Source: CAD feature listing. Evaluate the final solid. Frame: model axes, mm. Face numbers are marked on the shaded views. A direction names the side the tool comes from. Round coordinates to 2 decimals unless told otherwise and drop trailing zeros. Loops run counter-clockwise (first coordinate to the right, second up) from the corner with the lowest first, then second, coordinate; pieces in that order, holes last. Notation, with made-up numbers: (85.25, 42) -> (97.25, 42) arc R19 cw to (97.25, 72) -> close; hole circle Ø9 at (-2, -27). An arc over 180 degrees is marked (long way). Put each result on its own line as item: value. Start each with the question number.
1. Cut plane D-D (x = -65.5). Return the cut outline in (y, z), then the cut area to 3 significant figures.
2. Draft query along X for the marked faces 3, 4, 5 and 6. Return one class per face: pulls with the +X half, pulls with the -X half, needs draft (parallel to the pull), parting line crosses it, or undercut.
3. Contact query for flat-ended pins moving along their axis: pin 1 (8 mm diameter, centred on x = 70.5, z = 36, fed in from +Y); pin 2 (2 mm diameter, centred on y = 35.5, z = 20.5, fed in from -X); pin 3 (5 mm diameter, centred on y = 13.5, z = 41.25, fed in from -X). Output: stop coordinate, or through.
4. Cut plane A-A (y = 18). Return the cut outline in (x, z).
5. Cut plane C-C (y = 8.5). Return the cut outline in (x, z), then the cut area to 3 significant figures.
6. Cut plane B-B (x = 39). Return the cut outline in (y, z), then the cut area to 4 significant figures.
7. Material intervals for L1, parallel to Z at x = -115.2, y = 4.5; L2, parallel to Y at x = -14.5, z = 3; L3, parallel to X at y = 10.5, z = 25.5, sorted ascending.
8. Set-up query: the marked faces 1 and 2. Return all of +Z, -Z, +X, -X, +Y, -Y with unobstructed straight access to the full face (end or side cutting, diameter ignored); none if empty.
```python
from build123d import *

# Parameters (mm, degrees)
BOSS_EXTRUDE1_DEPTH     = 45
CUT_EXTRUDE1_DEPTH      = 7.5
SKETCH4_R               = 1.5
CUT_EXTRUDE2_DEPTH      = 7.5
CUT_EXTRUDE3_DEPTH      = 139.338353323
CUT_EXTRUDE3_DEPTH_BACK = 139.338353323
SKETCH5_R               = 1.5


with BuildPart() as part:
    # Sketch1 → Boss-Extrude1 (new body)
    with BuildSketch(Plane.XY):
        with BuildLine():
            ThreePointArc((-112.5, 0), (-97.123106012, 37.123106012), (-60, 52.5))
            Line((-60, 52.5), (60, 52.5))
            ThreePointArc((60, 52.5), (97.123106012, 37.123106012), (112.5, 0))
            Line((112.5, 0), (117.5, 0))
            ThreePointArc((117.5, 0), (100.658639918, 40.658639918), (60, 57.5))
            Line((60, 57.5), (-60, 57.5))
            ThreePointArc((-60, 57.5), (-100.658639918, 40.658639918), (-117.5, 0))
            Line((-117.5, 0), (-112.5, 0))
        make_face()
    extrude(amount=BOSS_EXTRUDE1_DEPTH)

    # Sketch3 → Cut-Extrude1 (cut)
    with BuildSketch(Plane.XY.offset(45)):
        with BuildLine():
            Line((-115.5, 0), (115.5, 0))
            ThreePointArc((115.5, 0), (99.244426356, 39.244426356), (60, 55.5))
            Line((60, 55.5), (-60, 55.5))
            ThreePointArc((-60, 55.5), (-99.244426356, 39.244426356), (-115.5, 0))
        make_face()
    extrude(amount=-CUT_EXTRUDE1_DEPTH, mode=Mode.SUBTRACT)

    # Sketch4 → Cut-Extrude2 (cut)
    with BuildSketch(Plane(origin=(0, 57.5, 0), x_dir=(1, 0, 0), z_dir=(0, 1, 0))):
        with Locations(Location((33, -3.75, 0), (0, 0, 270))):
            Circle(SKETCH4_R)
        with Locations(Location((11, -41.25, 0), (0, 0, 270))):
            Circle(SKETCH4_R)
        with Locations(Location((33, -41.25, 0), (0, 0, 270))):
            Circle(SKETCH4_R)
        with Locations(Location((55, -41.25, 0), (0, 0, 270))):
            Circle(SKETCH4_R)
        with Locations(Location((-33, -3.75, 0), (0, 0, 180))):
            Circle(SKETCH4_R)
        with Locations(Location((-11, -41.25, 0), (0, 0, 180))):
            Circle(SKETCH4_R)
        with Locations(Location((-33, -41.25, 0), (0, 0, 180))):
            Circle(SKETCH4_R)
        with Locations(Location((-55, -41.25, 0), (0, 0, 180))):
            Circle(SKETCH4_R)
    extrude(amount=-CUT_EXTRUDE2_DEPTH, mode=Mode.SUBTRACT)

    # Sketch5 → Cut-Extrude3 (cut, two sides: drawn at the far end of the back side and taken through both)
    with BuildSketch(Plane(origin=(0, 0, 0), x_dir=(0, 0, -1), z_dir=(1, 0, 0)).offset(-CUT_EXTRUDE3_DEPTH_BACK)):
        with Locations((-3.75, 4.5)):
            Circle(SKETCH5_R)
        with Locations((-41.25, 4.5)):
            Circle(SKETCH5_R)
        with Locations((-41.25, 13.5)):
            Circle(SKETCH5_R)
    extrude(amount=CUT_EXTRUDE3_DEPTH + CUT_EXTRUDE3_DEPTH_BACK, mode=Mode.SUBTRACT)


solid = part.part
```
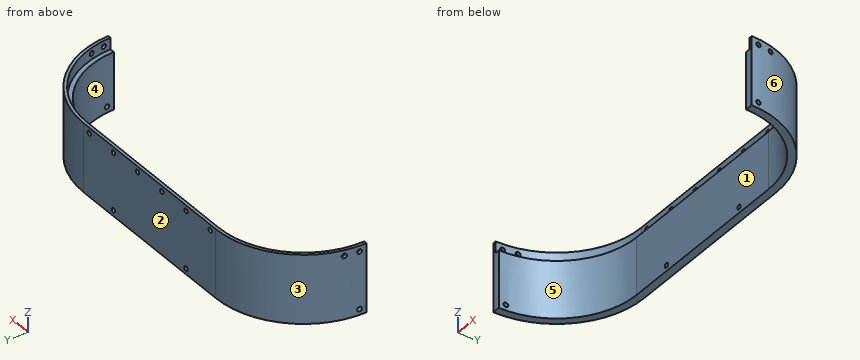
Solution:
1. outline: (52.21, 0) -> (57.24, 0) -> (57.24, 45) -> (55.23, 45) -> (55.23, 37.5) -> (52.21, 37.5) -> close
1. area: 204 mm^2
2. face 3: pulls with the -X half
2. face 4: undercut
2. face 5: undercut
2. face 6: pulls with the +X half
3. pin 1: stops at y = 57.13
3. pin 2: stops at x = -106
3. pin 3: stops at x = -116.44
4. outline: (-114.61, 0) -> (-109.32, 0) -> (-109.32, 37.5) -> (-112.5, 37.5) -> (-112.5, 45) -> (-114.61, 45) -> close; (109.32, 0) -> (114.61, 0) -> (114.61, 45) -> (112.5, 45) -> (112.5, 37.5) -> (109.32, 37.5) -> close
5. outline: (-116.87, 0) -> (-111.81, 0) -> (-111.81, 37.5) -> (-114.85, 37.5) -> (-114.85, 45) -> (-116.87, 45) -> close; (111.81, 0) -> (116.87, 0) -> (116.87, 45) -> (114.85, 45) -> (114.85, 37.5) -> (111.81, 37.5) -> close
5. area: 410 mm^2
6. outline: (52.5, 0) -> (57.5, 0) -> (57.5, 45) -> (55.5, 45) -> (55.5, 37.5) -> (52.5, 37.5) -> close
6. area: 202.5 mm^2
7. L1: z = 0 to 2.25, 5.25 to 37.5
7. L2: y = 52.5 to 57.5
7. L3: x = -116.53 to -111.44, 111.44 to 116.53
8. face 1: +Z, -Z, -Y
8. face 2: +Z, -Z, +X, -X, +Y
